Autodesk Inventor part; units mm, degrees
ref_plane "YZ Plane" through (0, 0, 0) normal (1, 0, 0) x (0, 1, 0)
ref_plane "XZ Plane" through (0, 0, 0) normal (0, 1, 0) x (-1, 0, 0)
ref_plane "XY Plane" through (0, 0, 0) normal (0, 0, 1) x (1, 0, 0)
sketch "Sketch9" plane through (0, 0, 0) normal (0, 1, 0) x (-1, 0, 0)
  line L0 (30, 30) -> (-30, 30)
  line L1 (-30, 30) -> (-30, -30)
  line L2 (-30, -30) -> (30, -30)
  line L3 (30, -30) -> (30, 30)
  line L4 (30, 30) -> (-30, -30) construction
  line L5 (-30, 30) -> (30, -30) construction
  line L6 (-28, 28) -> (28, 28)
  line L7 (28, 28) -> (28, -28)
  line L8 (28, -28) -> (-28, -28)
  line L9 (-28, -28) -> (-28, 28)
  point P0 (0, 0)
  dimension "d172" = 60
  dimension "d173" = 60
  dimension "d174" = 2
extrude "Extrusion3" add sketch "Sketch9" against normal blind 150
properties part number "TZS 1762 FDS 940x50 column" material "Stainless Steel"
Check sheet for the modelled part. Datum: model origin and axes. Units: mm. A direction names the side the tool comes from. Give positions to 0.01 mm unless a question says otherwise; leave off trailing zeros. Loops run counter-clockwise (first coordinate to the right, second up) from the corner with the lowest first, then second, coordinate; pieces in that order, holes last. Notation, with made-up numbers: M 45.25,25.5 L 95.25,25.5 A11 ccw 95.25,40.5 Z; hole C -20,64 d10. An arc over 180 degrees is marked long. Answer in a Markdown table with one row per item.
1) Thickness scan on line 1 (Z direction, x = -23, y = -15). Record the ranges inside material, lowest first.
Solutions:
| item | result |
|---|---|
| line 1 | z = -30 to -28, 28 to 30 |
2) Cross-section at A-A (z = 6). Enter the section's corners in (x, y), plus the area to 3 significant figures.
Solutions:
| item | result |
|---|---|
| outline | M -30,-150 L -28,-150 L -28,0 L -30,0 Z; M 28,-150 L 30,-150 L 30,0 L 28,0 Z |
| area | 600 mm^2 |
3) Cross-section at B-B (y = -95). Enter the section's corners in (x, z).
Solutions:
| item | result |
|---|---|
| outline | M -30,-30 L 30,-30 L 30,30 L -30,30 Z; hole M -28,-28 L 28,-28 L 28,28 L -28,28 Z |
4) Cross-section at C-C (x = 15). Enter the section's corners in (y, z).
Solutions:
| item | result |
|---|---|
| outline | M -150,-30 L 0,-30 L 0,-28 L -150,-28 Z; M -150,28 L 0,28 L 0,30 L -150,30 Z |
5) Mould release check, pull along Z, two halves, no side actions. Record for faces 1 (the face through (2, 0, -29)), 2 (the face through (0, -74, 30)), 3 (the face through (0, -74, 28)): released by +Z, released by -Z, zero draft, split by the parting line, or undercut.
Solutions:
| item | result |
|---|---|
| face 1 | zero draft |
| face 2 | released by +Z |
| face 3 | undercut |
6) Tool access check on faces 4 (the face through (0, -74, -28)), 5 (the face through (-30, -74, 0)). Record the directions out of +Z, -Z, +X, -X, +Y, -Y that give a thin tool (end or side, any length) a straight path to the whole face; none if there is none.
Solutions:
| item | result |
|---|---|
| face 4 | +Y, -Y |
| face 5 | +Z, -Z, -X, +Y, -Y |
